Input: part model. Units: mm. Frame: model coordinates. Face numbers are marked on the shaded views. A direction names the side the tool comes from. Coordinates: 2 decimals unless noted, no trailing zeros. Write each loop counter-clockwise with the first axis right and the second up, starting at its lowest first coordinate (ties: lowest second). Pieces come first, ordered by that corner, then holes. Notation, with made-up numbers: (46, 47) - (95, 47) arc R29 ccw to (95, 83) - close; hole circle Ø9 at (22.5, -34.5). An arc over 180 degrees is marked (long way). One line per question, with ' | ' between items. Start each with the question number.
1) Line query: line 1 (Z direction, x = 170, y = -25.5); line 2 (Z direction, x = 95, y = -35.5); line 3 (Y direction, x = 196, z = 15.5). Output: solid intervals per line, ascending.
2) First-contact query: P1, Ø5, axis at x = 135.5, z = -14, coming from the -Y side; P2, Ø8, axis at x = 183, z = -5, coming from the -Y side; P3, Ø16, axis at x = 172, z = 6, coming from the -Y side. Flat tips, straight axial feed; report the tip coordinate or a pass-through.
3) Reachability of the marked faces 1 and 2 from +Z, -Z, +X, -X, +Y, -Y: full face, straight path, thin tool, end or side. Return the list, or none.
4) Section query A-A on y = -10.5. Return loops of the section in (x, z), and give its area (3 significant figures).
5) Draft query along Z for the marked faces 3, 4 and 5. Return one class per face: released by +Z, released by -Z, zero draft, split by the parting line, or undercut.
6) Section query B-B on x = 171. Return loops of the section in (y, z).
7) Section query C-C on z = 8.5. Return loops of the section in (x, y), and give its area (4 significant figures).
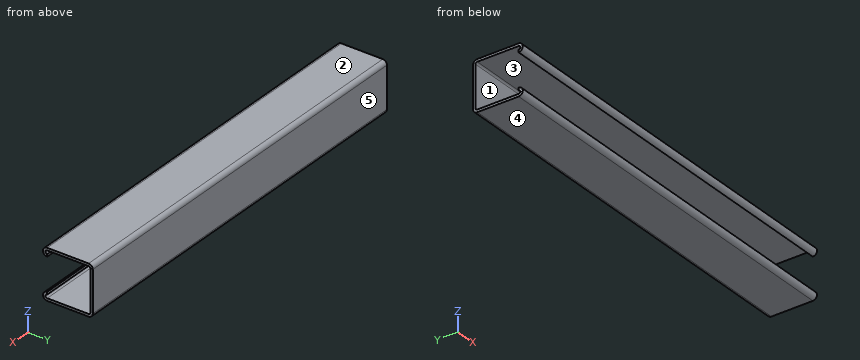
```python
from build123d import *

# Parameters (mm, degrees)
CHANNEL_DEPTH = 305


with BuildPart() as part:
    # Sketch1 → Channel (new body)
    with BuildSketch(Plane(origin=(0, 39.243400922, 0), x_dir=(0, 0, 1), z_dir=(1, 0, 0))):
        with BuildLine():
            ThreePointArc((-12.65, 74.143400922), (-15.85, 77.343400922), (-19.05, 74.143400922))
            Line((-19.05, 74.143400922), (-19.05, 42.443400922))
            ThreePointArc((-19.05, 42.443400922), (-18.1127417, 40.180659222), (-15.85, 39.243400922))
            Line((-15.85, 39.243400922), (15.85, 39.243400922))
            ThreePointArc((15.85, 39.243400922), (18.1127417, 40.180659222), (19.05, 42.443400922))
            Line((19.05, 42.443400922), (19.05, 74.143400922))
            ThreePointArc((19.05, 74.143400922), (15.85, 77.343400922), (12.65, 74.143400922))
            Line((12.65, 74.143400922), (14.55, 74.143400922))
            ThreePointArc((14.55, 74.143400922), (15.85, 75.443400922), (17.15, 74.143400922))
            Line((17.15, 74.143400922), (17.15, 42.443400922))
            ThreePointArc((17.15, 42.443400922), (16.769238816, 41.524162106), (15.85, 41.143400922))
            Line((15.85, 41.143400922), (-15.85, 41.143400922))
            ThreePointArc((-15.85, 41.143400922), (-16.769238816, 41.524162106), (-17.15, 42.443400922))
            Line((-17.15, 42.443400922), (-17.15, 74.143400922))
            ThreePointArc((-17.15, 74.143400922), (-15.85, 75.443400922), (-14.55, 74.143400922))
            Line((-14.55, 74.143400922), (-12.65, 74.143400922))
        make_face()
    extrude(amount=CHANNEL_DEPTH)


solid = part.part
```
Answer key:
1) line 1: -19.05 to -17.15, 17.15 to 19.05 | line 2: -18.99 to -17, -14.7 to -12.71, 12.71 to 14.7, 17 to 18.99 | line 3: -38.08 to -36.15, -1.9 to 0
2) P1: y = -38.1 | P2: y = -1.9 | P3: y = -37.51
3) face 1: +X, -X | face 2: +Z, +X, -X, +Y, -Y
4) outline: (0, -19.05) - (305, -19.05) - (305, -17.15) - (0, -17.15) - close; (0, 17.15) - (305, 17.15) - (305, 19.05) - (0, 19.05) - close | area: 1,160 mm²
5) face 3: undercut | face 4: released by -Z | face 5: zero draft
6) outline: (-34.9, -19.05) - (-3.2, -19.05) arc R3.2 ccw to (0, -15.85) - (0, 15.85) arc R3.2 ccw to (-3.2, 19.05) - (-34.9, 19.05) arc R3.2 ccw to (-34.9, 12.65) - (-34.9, 14.55) arc R1.3 cw to (-34.9, 17.15) - (-3.2, 17.15) arc R1.3 cw to (-1.9, 15.85) - (-1.9, -15.85) arc R1.3 cw to (-3.2, -17.15) - (-34.9, -17.15) arc R1.3 cw to (-34.9, -14.55) - (-34.9, -12.65) arc R3.2 ccw to start
7) outline: (0, -1.9) - (305, -1.9) - (305, 0) - (0, 0) - close | area: 579.5 mm²
